Source: CAD feature listing. Evaluate the final solid. Frame: model axes, mm. A direction names the side the tool comes from. Coordinates: 2 decimals unless noted, no trailing zeros. Write each loop counter-clockwise with the first axis right and the second up, starting at its lowest first coordinate (ties: lowest second). Pieces come first, ordered by that corner, then holes. Notation, with made-up numbers: M 23.5,89 L 61.5,89 A30 cw 61.5,112 Z; hole C 53.25,42 d3. An arc over 180 degrees is marked long. Answer as CSV lines item,"result". Start each with the question number.
1. Section B-B on x = -0.75. Return the cut outline in (y, z), plus the area to 3 significant figures.
2. Contact query for flat-ended pins moving along their axis: pin 1 Ø1.8 at (x, z) = (0, 80) entering from +Y; pin 2 Ø4 at (x, y) = (-2, 4) entering from +Z. Output: stop coordinate, or through.
3. Mould query, pull axis Y, two halves, no side actions, for faces 1 (the face through (0, -4, 50)), 2 (the face through (-0.195, -4.507, 18.164)), 3 (the face through (0, -5, 50)), 4 (the face through (-4, 0, 50)). Classes: pulls with the +Y half, pulls with the -Y half, needs draft (parallel to the pull), parting line crosses it, or undercut.
4. Section C-C on z = 80. Return the cut outline in (x, y), plus the area to 3 significant figures.
5. Section D-D on z = 62. Return the cut outline in (x, y), plus the area to 3 significant figures.
6. Reachability of faces 5 (the face through (4, 0, 51)), 6 (the face through (-0.195, 4.493, 18.164)) from +Z, -Z, +X, -X, +Y, -Y: full face, straight path, thin tool, end or side. Return the list, or none.
7. Line query: probe 1 along X at (y, z) = (-2.75, 81); probe 2 along Z at (x, y) = (0, 4.55). Output: solid intervals per line, ascending. Write a range as [from, to].
8. Section A-A on y = 3.25. Return the cut outline in (x, z).
```python
from build123d import *

# Parameters (mm, degrees)
SKETCH_1_W          = 10
SKETCH_1_H          = 10
SKETCH_1_W_2        = 8
SKETCH_1_H_2        = 8
EXTRUDE_1_DEPTH     = 90
SKETCH_2_R          = 1.5
CUT_EXTRUDE_1_DEPTH = 11


with BuildPart() as part:
    # 草图1 → 拉伸-薄壁1 (new body)
    with BuildSketch(Plane.XY):
        Rectangle(SKETCH_1_W, SKETCH_1_H)
        Rectangle(SKETCH_1_W_2, SKETCH_1_H_2, mode=Mode.SUBTRACT)
    extrude(amount=EXTRUDE_1_DEPTH)

    # 草图2 → 切除-拉伸1 (cut, through all)
    with BuildSketch(Plane.XZ.offset(5)):
        Polygon((1.92820323, 12), (-5, 0), (5, 0), (5, 17.320508076), align=None)
        Polygon((-5, 12), (-5, 0), (1.92820323, 12), align=None)
        with Locations((0, 16.676515813)):
            Circle(SKETCH_2_R)
        Polygon((5, 90), (-5, 90), (5, 87.320508076), align=None)
        with Locations((0, 80)):
            Circle(SKETCH_2_R)
    extrude(amount=-CUT_EXTRUDE_1_DEPTH, mode=Mode.SUBTRACT)


solid = part.part
```
Values:
1,outline,"M -5,12 L -4,12 L -4,15.38 L -5,15.38 Z; M -5,17.98 L -4,17.98 L -4,78.7 L -5,78.7 Z; M -5,81.3 L -4,81.3 L -4,88.86 L -5,88.86 Z; M 4,12 L 5,12 L 5,15.38 L 4,15.38 Z; M 4,17.98 L 5,17.98 L 5,78.7 L 4,78.7 Z; M 4,81.3 L 5,81.3 L 5,88.86 L 4,88.86 Z"
1,area,"143 mm²"
2,pin 1,"through"
2,pin 2,"z = 89.73"
3,face 1,"undercut"
3,face 2,"needs draft"
3,face 3,"pulls with the -Y half"
3,face 4,"undercut"
4,outline,"M -5,-5 L -1.5,-5 L -1.5,-4 L -4,-4 L -4,4 L -1.5,4 L -1.5,5 L -5,5 Z; M 1.5,-5 L 5,-5 L 5,5 L 1.5,5 L 1.5,4 L 4,4 L 4,-4 L 1.5,-4 Z"
4,area,"30.0 mm²"
5,outline,"M -5,-5 L 5,-5 L 5,5 L -5,5 Z; hole M -4,-4 L 4,-4 L 4,4 L -4,4 Z"
5,area,"36.0 mm²"
6,face 5,"+Z, -Z"
6,face 6,"+Y, -Y"
7,probe 1,"[-5, -4], [4, 5]"
7,probe 2,"[12, 15.18], [18.18, 78.5], [81.5, 88.66]"
8,outline,"M -5,12 L -4,12 L -4,89.73 L -5,90 Z; M 4,15.59 L 5,17.32 L 5,87.32 L 4,87.59 Z"
